from build123d import *

# Parameters (mm, degrees)
SKETCH_1_W          = 95
SKETCH_1_H          = 38.85
EXTRUDE_1_DEPTH     = 0.5
SKETCH_2_W          = 38.85
SKETCH_2_H          = 95
EXTRUDE_2_DEPTH     = 0.5
CUT_EXTRUDE_1_DEPTH = 110.347085009


with BuildPart() as part:
    # Эскиз1 → Бобышка-Вытянуть1 (new body)
    with BuildSketch(Plane(origin=(0.5, 0, 0), x_dir=(0, -1, 0), z_dir=(-1, 0, 0))):
        with Locations((-53.35, 22.825)):
            Rectangle(SKETCH_1_W, SKETCH_1_H)
    extrude(amount=-EXTRUDE_1_DEPTH)

    # Эскиз2 → Бобышка-Вытянуть2 (add)
    with BuildSketch(Plane.ZY.offset(-0.5)):
        with Locations((22.825, 53.35)):
            Rectangle(SKETCH_2_W, SKETCH_2_H)
    extrude(amount=EXTRUDE_2_DEPTH)

    # Эскиз3 → Вырез-Вытянуть1 (cut, through all)
    with BuildSketch(Plane.ZY):
        Polygon((47.187175015, 54.261978396), (29.562288031, 54.261978396), (29.562288031, 50.078726521), (28.618889228, 50.078726521), (28.618889228, 47.878726521), (29.562288031, 47.878726521), (29.562288031, 33.238726521), (28.618889228, 33.238726521), (28.618889228, 31.038726521), (29.562288031, 31.038726521), (29.562288031, 25.969159943), (47.187175015, 25.969159943), align=None)
    extrude(amount=-CUT_EXTRUDE_1_DEPTH, mode=Mode.SUBTRACT)


solid = part.part
Here's how the part is built. I have some questions about the finished solid (model axes, mm). Coordinates: 2 decimals unless noted, no trailing zeros. Order: outer loops, then holes, each group sorted by start corner. A loop starts at its lowest first (then second) coordinate and runs counter-clockwise, first axis right, second up.
Item 1: If we section it at A-A on z = 39.5: List the corners of the cut face in (x, y) for me.
Result sheet:
outline: (0, 5.85) - (1, 5.85) - (1, 25.97) - (0, 25.97) - close; (0, 54.26) - (1, 54.26) - (1, 100.85) - (0, 100.85) - close
Item 2: If we section it at C-C on y = 36: List the corners of the cut face in (x, z) for me, plus the area to 3 significant figures.
Result sheet:
outline: (0, 3.4) - (1, 3.4) - (1, 29.56) - (0, 29.56) - close
area: 26.2 mm2
Item 3: If we section it at B-B on x = 0.6: List the corners of the cut face in (y, z) for me.
Result sheet:
outline: (5.85, 3.4) - (100.85, 3.4) - (100.85, 42.25) - (54.26, 42.25) - (54.26, 29.56) - (50.08, 29.56) - (50.08, 28.62) - (47.88, 28.62) - (47.88, 29.56) - (33.24, 29.56) - (33.24, 28.62) - (31.04, 28.62) - (31.04, 29.56) - (25.97, 29.56) - (25.97, 42.25) - (5.85, 42.25) - close
Item 4: I need wall thicknesses on line 1 (Y direction, x = 0.45, z = 39); line 2 (Z direction, x = 0.6, y = 41). Which ranges of each line are inside material? Lowest first, please.
Result sheet:
line 1: y = 5.85 to 25.97, 54.26 to 100.85
line 2: z = 3.4 to 29.56
